from build123d import *

# Parameters (mm, degrees)
F0_R     = 3.81
F1_DEPTH = 4
F2_DEPTH = 12.7
F3_DEPTH = 10


# Not quite as in the source:
# - a feature names something its author has since deleted; it is built from what else it names


with BuildPart() as f1:
    # F0 (on Top) → F1 (new body)
    with BuildSketch(Plane.XY):
        with BuildLine():
            ThreePointArc((6.7162400934, 21.1859090909), (14.3680496868, 16.9561131513), (19.7963307394, 10.1022727273))
            Line((19.7963307394, 10.1022727273), (8.4841417455, 32.2695454545))
            ThreePointArc((8.4841417455, 32.2695454545), (9.2611304689, 30.1664517595), (9.525, 27.94))
            ThreePointArc((9.525, 27.94), (8.7948226784, 24.2825802736), (6.7162400934, 21.1859090909))
        make_face()
        with BuildLine():
            Line((-8.4841417455, 32.2695454545), (-19.7963307394, 10.1022727273))
            ThreePointArc((-19.7963307394, 10.1022727273), (-14.3680496868, 16.9561131513), (-6.7162400934, 21.1859090909))
            ThreePointArc((-6.7162400934, 21.1859090909), (-9.4060964683, 26.4396752924), (-8.4841417455, 32.2695454545))
        make_face()
        with BuildLine():
            ThreePointArc((-19.7963307394, 10.1022727273), (-5.1950541054, -21.6093044275), (22.225, 0))
            ThreePointArc((22.225, 0), (21.6093044275, 5.1950541054), (19.7963307394, 10.1022727273))
            ThreePointArc((19.7963307394, 10.1022727273), (14.3680496868, 16.9561131513), (6.7162400934, 21.1859090909))
            ThreePointArc((6.7162400934, 21.1859090909), (0, 18.415), (-6.7162400934, 21.1859090909))
            ThreePointArc((-6.7162400934, 21.1859090909), (-14.3680496868, 16.9561131513), (-19.7963307394, 10.1022727273))
        make_face()
        with BuildLine():
            ThreePointArc((-6.7162400934, 21.1859090909), (0, 22.225), (6.7162400934, 21.1859090909))
            ThreePointArc((6.7162400934, 21.1859090909), (8.7948226784, 24.2825802736), (9.525, 27.94))
            ThreePointArc((9.525, 27.94), (9.2611304689, 30.1664517595), (8.4841417455, 32.2695454545))
            ThreePointArc((8.4841417455, 32.2695454545), (0, 37.465), (-8.4841417455, 32.2695454545))
            ThreePointArc((-8.4841417455, 32.2695454545), (-9.4060964683, 26.4396752924), (-6.7162400934, 21.1859090909))
        make_face()
        with Locations((0, 27.94)):
            Circle(F0_R, mode=Mode.SUBTRACT)
        with BuildLine():
            ThreePointArc((-6.7162400934, 21.1859090909), (0, 18.415), (6.7162400934, 21.1859090909))
            ThreePointArc((6.7162400934, 21.1859090909), (0, 22.225), (-6.7162400934, 21.1859090909))
        make_face()
    extrude(amount=F1_DEPTH)

    # F0 (on Top) → F2 (join)
    with BuildSketch(Plane.XY):
        with BuildLine():
            ThreePointArc((-19.7963307394, 10.1022727273), (-5.1950541054, -21.6093044275), (22.225, 0))
            ThreePointArc((22.225, 0), (21.6093044275, 5.1950541054), (19.7963307394, 10.1022727273))
            ThreePointArc((19.7963307394, 10.1022727273), (14.3680496868, 16.9561131513), (6.7162400934, 21.1859090909))
            ThreePointArc((6.7162400934, 21.1859090909), (0, 18.415), (-6.7162400934, 21.1859090909))
            ThreePointArc((-6.7162400934, 21.1859090909), (-14.3680496868, 16.9561131513), (-19.7963307394, 10.1022727273))
        make_face()
        with BuildLine():
            ThreePointArc((-6.7162400934, 21.1859090909), (0, 18.415), (6.7162400934, 21.1859090909))
            ThreePointArc((6.7162400934, 21.1859090909), (0, 22.225), (-6.7162400934, 21.1859090909))
        make_face()
    extrude(amount=F2_DEPTH)

    # F0 (on Top) → F3 (join)
    with BuildSketch(Plane.XY):
        with BuildLine():
            ThreePointArc((-6.7162400934, 21.1859090909), (0, 18.415), (6.7162400934, 21.1859090909))
            ThreePointArc((6.7162400934, 21.1859090909), (0, 22.225), (-6.7162400934, 21.1859090909))
        make_face()
        with BuildLine():
            ThreePointArc((-19.7963307394, 10.1022727273), (-5.1950541054, -21.6093044275), (22.225, 0))
            ThreePointArc((22.225, 0), (21.6093044275, 5.1950541054), (19.7963307394, 10.1022727273))
            ThreePointArc((19.7963307394, 10.1022727273), (14.3680496868, 16.9561131513), (6.7162400934, 21.1859090909))
            ThreePointArc((6.7162400934, 21.1859090909), (0, 18.415), (-6.7162400934, 21.1859090909))
            ThreePointArc((-6.7162400934, 21.1859090909), (-14.3680496868, 16.9561131513), (-19.7963307394, 10.1022727273))
        make_face()
    extrude(amount=F3_DEPTH)


solid = f1.part
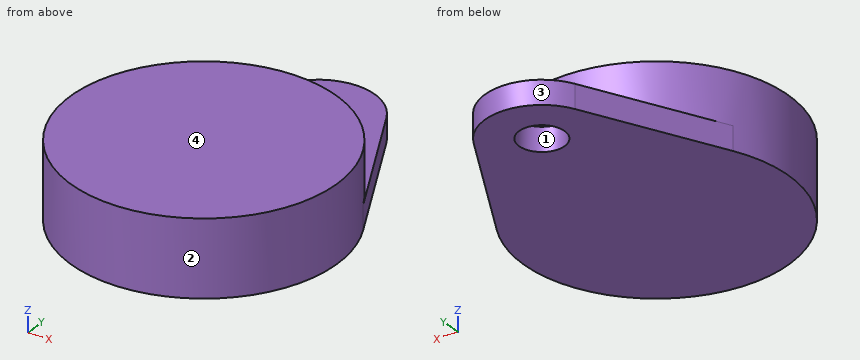
Could you check a few things on this model? Use its own coordinates, in mm. Face numbers are marked on the shaded views. Round coordinates to 2 decimals unless told otherwise and drop trailing zeros. Loops run counter-clockwise (first coordinate to the right, second up) from the corner with the lowest first, then second, coordinate; pieces in that order, holes last. Notation, with made-up numbers: (28, 70.25) - (76, 70.25) arc R16 cw to (76, 90.25) - close; hole circle Ø4 at (-35, 23). An arc over 180 degrees is marked (long way). Write item = value, one per line.
1) Imagine slicing it at B-B (z = 1). Please give me the cut outline in (x, y) (3 decimals).
Computed:
outline = (-19.796, 10.102) arc R22.225 ccw (long way) to (19.796, 10.102) - (8.484, 32.27) arc R9.525 ccw to (-8.484, 32.27) - close; hole circle Ø7.62 at (0, 27.94)
2) Imagine slicing it at A-A (x = 0). Please give me the cut outline in (y, z) (3 decimals).
Computed:
outline = (-22.225, 0) - (24.13, 0) - (24.13, 4) - (22.225, 4) - (22.225, 12.7) - (-22.225, 12.7) - close; (31.75, 0) - (37.465, 0) - (37.465, 4) - (31.75, 4) - close
3) Imagine slicing it at C-C (y = 27.94). Please give me the cut outline in (x, z), and give its area (3 significant figures).
Computed:
outline = (-10.69, 0) - (-3.81, 0) - (-3.81, 4) - (-10.69, 4) - close; (3.81, 0) - (10.69, 0) - (10.69, 4) - (3.81, 4) - close
area = 55.1 mm2
4) Imagine slicing it at D-D (z = 7.75). Please give me the cut outline in (x, y) (3 decimals).
Computed:
outline = circle Ø44.45 at (0, 0)
5) If we mould it in two halves opening along Y, with no side actions, what happens to the marked faces 1, 2, 3 and 4? For each: pulls with the +Y half, pulls with the -Y half, needs draft (parallel to the pull), parting line crosses it, or undercut.
Computed:
face_1 = undercut
face_2 = parting line crosses it
face_3 = pulls with the +Y half
face_4 = needs draft
6) I'm going to push flat-ended pins straight in: P1, Ø1, axis at x = 16, z = 8, coming from the -Y side; P2, Ø5, axis at x = -13.5, z = 8, coming from the -Y side; P3, Ø2, axis at y = -8.5, z = 5.5, coming from the -X side. Where does each tip first touch, or does it pass through?
Computed:
P1 = -15.93
P2 = -19.31
P3 = -20.92
7) I need wall thicknesses on line 1 along Y through (x, z) = (0, 2.2) (3 decimals); line 2 along Z through (x, y) = (-4.5, 30); line 3 along X through (y, z) = (0, 4.75) (3 decimals). Which ranges of each line are inside material? Lowest first, please. Write a range as from..to.
Computed:
line_1 = -22.225..24.13, 31.75..37.465
line_2 = 0..4
line_3 = -22.225..22.225
